Design review of the part built by this model. Coordinates are the model's own, in mm. A direction names the side the tool comes from. Coordinates: 2 decimals unless noted, no trailing zeros. Order: outer loops, then holes, each group sorted by start corner. A loop starts at its lowest first (then second) coordinate and runs counter-clockwise, first axis right, second up. Notation, with made-up numbers: M 55,13.25 L 78,13.25 A19 ccw 78,42.25 Z; hole C 48.25,-14.75 d9. An arc over 180 degrees is marked long. Answer in a Markdown table with one row per item.
Autodesk Inventor part; units mm, degrees
ref_plane "Work Plane1" through (0, -4, 9.6) normal (1, 0, 0) x (0, 0, -1)
ref_plane "YZ Plane" through (0, 0, 0) normal (1, 0, 0) x (0, 1, 0)
ref_plane "XZ Plane" through (0, 0, 0) normal (0, 1, 0) x (-1, 0, 0)
sketch "Sketch1" plane through (0, 0, 0) normal (0, 0, 1) x (1, 0, 0)
  line L0 (-4, -4) -> (4, -4)
  line L1 (4, -4) -> (4, 4)
  line L2 (4, 4) -> (-4, 4)
  line L3 (-4, 4) -> (-4, -4)
  line L4 (-4, -4) -> (4, 4) construction
  line L5 (4, -4) -> (-4, 4) construction
  circle A0 centre (0, 0) radius 2.4
  dimension "d0" = 8
  dimension "d1" = 8
  dimension "d2" = 4.8
extrude "Extrusion1" add sketch "Sketch1" along normal blind 9.6 contours L3 L2 L1 L0 | A0
extrude "Extrusion2" add sketch "Sketch1" along normal blind 11.3 contours A0
extrude "Extrusion3" cut sketch "Sketch1" along normal blind 1.7 contours A0
pattern_linear "Rectangular Pattern1" count 8 spacing 8 along (0, 1, 0) of "Extrusion1", "Extrusion2", "Extrusion3"
sketch "Sketch2" plane through (4, -4, 9.6) normal (1, 0, 0) x (0, 0, -1)
  circle A0 centre (4, 8) radius 2.4
  circle A1 centre (4, 8) radius 3.1
  line L0 (9.6, 0) -> (9.6, 64)
  line L1 (9.6, 0) -> (0, 0)
  point P0 (9.6, 4)
  dimension "d12" = 4.8
  dimension "d14" = 6.2
  dimension "d22" = 8
  dimension "d23" = 5.6
ref_plane "Work Plane1" through (0, -4, 9.6) normal (1, 0, 0) x (0, 0, -1)
extrude "Extrusion4" cut sketch "Sketch2" against normal up to next contours A0
extrude "Extrusion5" cut sketch "Sketch2" against normal blind 0.8
mirror "Mirror1" about plane through (0, -4, 9.6) normal (1, 0, 0) of "Extrusion5"
pattern_linear "Rectangular Pattern2" count 7 spacing 8 along (0, 1, 0) of "Extrusion4", "Extrusion5", "Mirror1"
equation "\"d11\" = d0"
equation "\"d21\" = d0"
properties part number "LEGO Technic Brick 1x8 with Holes"
(1) Add section B-B, the plane y = 4. Give the boundary of the cut face in (x, z), and give its area (3 significant figures).
Return value:
| item | result |
|---|---|
| outline | M -4,0 L 4,0 L 4,2.5 L 3.2,2.5 L 3.2,3.2 L -3.2,3.2 L -3.2,2.5 L -4,2.5 Z; M -4,8.7 L -3.2,8.7 L -3.2,8 L 3.2,8 L 3.2,8.7 L 4,8.7 L 4,9.6 L -4,9.6 Z |
| area | 36.2 mm2 |
(2) Insertion check: pin 1 Ø5 at (y, z) = (20, 5.6) entering from +X; pin 2 Ø5 at (y, z) = (4, 5.6) entering from -X; pin 3 Ø4 at (x, y) = (0, 24) entering from -Z. Each pin has a flat end and moves straight along its axis. Give the tip position at first contact, or say it passes through.
Return value:
| item | result |
|---|---|
| pin 1 | stops at x = 3.2 |
| pin 2 | stops at x = -3.2 |
| pin 3 | stops at z = 1.7 |
(3) Add section D-D, the plane x = -1.5. Give the number of separate pieces and of enclosed holes in the cut face, and give its area (3 significant figures).
Return value:
| item | result |
|---|---|
| separate pieces | 1 |
| enclosed holes | 7 |
| area | 488 mm2 |
(4) Draft analysis for pull direction Z (two halves, no side actions). For faces 1 (the flat face through (0, 16, 11.3)), 2 (the flat face through (0, 8, 1.7)), 3 (the flat face through (3.2, 18, 4)), state which applies: pulls with the +Z half, pulls with the -Z half, needs draft (parallel to the pull), parting line crosses it, or undercut.
Return value:
| item | result |
|---|---|
| face 1 | pulls with the +Z half |
| face 2 | pulls with the -Z half |
| face 3 | undercut |
(5) For line 1 along Z through (x, y) = (2.25, 45); line 2 along Z through (x, y) = (-0.25, 23.5); line 3 along Z through (x, y) = (3.5, 29), list the stretches that pass through material, from the lowest coordinate up. Write a range as from..to.
Return value:
| item | result |
|---|---|
| line 1 | z = 0..3.42, 7.78..9.6 |
| line 2 | z = 1.7..11.3 |
| line 3 | z = 0..2.67, 8.53..9.6 |
(6) For faces 4 (the cylindrical face through (3.61, 30.61, 3.93)), 5 (the flat face through (-3.2, 27, 3)), 6 (the cylindrical face through (-0.52, 26.343, 0.838)), list the 3-axis set-ups (+Z, -Z, +X, -X, +Y, -Y) from which the entire face can be reached by the end or side of a thin tool; tool diameter is ignored.
Return value:
| item | result |
|---|---|
| face 4 | +X |
| face 5 | -X |
| face 6 | -Z |
(7) Add section C-C, the plane y = 48. Give the boundary of the cut face in (x, z).
Return value:
| item | result |
|---|---|
| outline | M -4,0 L -2.4,0 L -2.4,1.7 L 2.4,1.7 L 2.4,0 L 4,0 L 4,9.6 L 2.4,9.6 L 2.4,11.3 L -2.4,11.3 L -2.4,9.6 L -4,9.6 Z |
(8) Add section A-A, the plane z = 10.5. Give the boundary of the cut face in (x, y).
Return value:
| item | result |
|---|---|
| outline | C 0,0 d4.8; C 0,8 d4.8; C 0,16 d4.8; C 0,24 d4.8; C 0,32 d4.8; C 0,40 d4.8; C 0,48 d4.8; C 0,56 d4.8 |
